Autodesk Inventor part; units mm, degrees
ref_plane "YZ Plane" through (0, 0, 0) normal (1, 0, 0) x (0, 1, 0)
ref_plane "XZ Plane" through (0, 0, 0) normal (0, 1, 0) x (-1, 0, 0)
ref_plane "XY Plane" through (0, 0, 0) normal (0, 0, 1) x (1, 0, 0)
sketch "Sketch2" plane through (0, 0, 0) normal (0, 1, 0) x (-1, 0, 0)
  line L0 (1.6384, 12.2587) -> (39.6384, 12.2587)
  line L1 (49.6384, 5.2687) -> (49.6384, -15.7313)
  line L2 (40.6384, -24.2313) -> (0.6384, -24.2313)
  line L3 (-8.3616, -15.7313) -> (-8.3616, 5.2687)
  line L4 (1.6384, 12.2587) -> (39.6384, 12.2587)
  line L5 (20.6384, 12.2587) -> (1.6384, 12.2587)
  line L6 (1.6384, 12.2587) -> (1.6384, 5.2687)
  line L7 (20.6384, 12.2587) -> (39.6384, 12.2587)
  line L8 (39.6384, 12.2587) -> (39.6384, 5.2687)
  circle A0 centre (31.1384, -0.7313) radius 4
  circle A1 centre (31.1384, 6.2687) radius 1.5
  circle A2 centre (24.1384, -0.7313) radius 1.5
  circle A3 centre (31.1384, -7.7313) radius 1.5
  circle A4 centre (38.1384, -0.7313) radius 1.5
  line L9 (31.1384, -0.7313) -> (40.1384, -0.7313) construction
  circle A5 centre (20.6384, -10.7313) radius 4
  circle A6 centre (20.6384, -3.7313) radius 1.5
  circle A7 centre (13.6384, -10.7313) radius 1.5
  circle A8 centre (20.6384, -17.7313) radius 1.5
  circle A9 centre (27.6384, -10.7313) radius 1.5
  line L10 (20.6384, -10.7313) -> (30.6384, -10.7313) construction
  line L11 (20.6384, 0) -> (20.6384, 3.2687)
  circle A10 centre (10.1384, -0.7313) radius 4
  circle A11 centre (10.1384, 6.2687) radius 1.5
  circle A12 centre (17.1384, -0.7313) radius 1.5
  circle A13 centre (10.1384, -7.7313) radius 1.5
  circle A14 centre (3.1384, -0.7313) radius 1.5
  line L12 (10.1384, -0.7313) -> (1.1384, -0.7313) construction
  line L13 (1.6384, 5.2687) -> (1.6384, 1.7687)
  line L14 (1.6384, 1.7687) -> (0.6384, 1.7687)
  line L15 (0.6384, 1.7687) -> (0.6384, 5.2687)
  line L16 (39.6384, 5.2687) -> (39.6384, 1.7687)
  line L17 (39.6384, 1.7687) -> (40.6384, 1.7687)
  line L18 (40.6384, 1.7687) -> (40.6384, 5.2687)
  circle A15 centre (-3.8616, -1.2313) radius 2
  circle A16 centre (-3.8616, -11.2313) radius 2
  line L19 (0.6384, 5.2687) -> (0.6384, 6.2687)
  line L20 (0.6384, 6.2687) -> (-8.3616, 6.2687)
  line L21 (-8.3616, 6.2687) -> (-8.3616, 5.2687)
  line L22 (40.6384, 5.2687) -> (40.6384, 6.2687)
  line L23 (40.6384, 6.2687) -> (49.6384, 6.2687)
  line L24 (49.6384, 6.2687) -> (49.6384, 5.2687)
  circle A17 centre (45.1384, -1.2313) radius 2
  circle A18 centre (45.1384, -11.2313) radius 2
  line L25 (0.6384, -24.2313) -> (0.6384, -17.7313)
  line L26 (0.6384, -17.7313) -> (-6.3616, -17.7313)
  line L27 (40.6384, -24.2313) -> (40.6384, -17.7313)
  line L28 (40.6384, -17.7313) -> (47.6384, -17.7313)
  arc A19 (-8.3616, -15.7313) -> (-6.3616, -17.7313) centre (-6.3616, -15.7313) ccw
  arc A20 (47.6384, -17.7313) -> (49.6384, -15.7313) centre (47.6384, -15.7313) ccw
  line L29 (1.6384, 12.2587) -> (39.6384, 12.2587)
  line L30 (40.6384, -24.2313) -> (1.6384, -24.2313)
  line L31 (1.6384, 1.7687) -> (1.6384, 12.2587)
  line L32 (40.6384, 6.2687) -> (40.6384, 1.7687)
  line L33 (40.6384, -17.7313) -> (40.6384, -24.2313)
  line L34 (49.6384, 6.2687) -> (49.6384, -15.7313)
  line L35 (-8.3616, -15.7313) -> (-8.3616, 6.2687)
  line L36 (40.6384, 6.2687) -> (49.6384, 6.2687)
  line L37 (-8.3616, 6.2687) -> (0.6384, 6.2687)
  line L38 (47.6384, -17.7313) -> (40.6384, -17.7313)
  line L39 (0.6384, -17.7313) -> (-6.3616, -17.7313)
  line L40 (-8.3616, 6.2687) -> (-8.3616, -15.7313)
  line L41 (-6.3616, -17.7313) -> (0.6384, -17.7313)
  line L42 (0.6384, -24.2313) -> (0.6384, -17.7313)
  line L43 (-6.3616, -17.7313) -> (0.6384, -17.7313)
  line L44 (0.6384, -24.2313) -> (40.6384, -24.2313)
  line L45 (40.6384, -24.2313) -> (40.6384, -17.7313)
  line L46 (40.6384, -17.7313) -> (47.6384, -17.7313)
  line L47 (49.6384, -15.7313) -> (49.6384, 6.2687)
  line L48 (49.6384, 6.2687) -> (40.6384, 6.2687)
  line L49 (40.6384, 6.2687) -> (40.6384, 1.7687)
  line L50 (39.6384, 1.7687) -> (40.6384, 1.7687)
  line L51 (39.6384, 1.7687) -> (39.6384, 12.2587)
  line L52 (39.6384, 12.2587) -> (1.6384, 12.2587)
  line L53 (1.6384, 12.2587) -> (1.6384, 1.7687)
  line L54 (1.6384, 1.7687) -> (0.6384, 1.7687)
  line L55 (0.6384, 1.7687) -> (0.6384, 6.2687)
  line L56 (0.6384, 6.2687) -> (-8.3616, 6.2687)
  line L57 (-8.3616, 6.2687) -> (-8.3616, -15.7313)
  point P0 (0, 0)
  dimension "d12" = 360
  dimension "d19" = 360
  dimension "d22" = 10
  dimension "d23" = 29
  dimension "d24" = 29
  dimension "d25" = 10.5
  dimension "d26" = 21
  dimension "d32" = 1
  dimension "d33" = 3.5
  dimension "d34" = 1
  dimension "d37" = 4
  dimension "d38" = 4
  dimension "d41" = 2
extrude "Extrusion1" add sketch "Sketch2" along normal blind 1
sketch "Sketch3" plane through (0, 1, 0) normal (0, 1, 0) x (1, 0, 0)
  line L0 (-0.6384, 17.7313) -> (-0.6384, 24.2313)
  line L1 (-49.6384, 15.7313) -> (-49.6384, -6.2687)
  line L2 (-0.6384, -1.7687) -> (-0.6384, -6.2687)
  line L3 (8.3616, -6.2687) -> (8.3616, 15.7313)
  line L4 (-40.6384, 24.2313) -> (-0.6384, 24.2313)
  line L5 (-0.6384, 24.2313) -> (-0.6384, 23.2313)
  line L6 (-0.6384, 23.2313) -> (-40.6384, 23.2313)
  line L7 (-40.6384, 23.2313) -> (-40.6384, 24.2313)
  line L8 (-0.6384, -6.2687) -> (8.3616, -6.2687)
  line L9 (8.3616, -6.2687) -> (8.3616, -5.2687)
  line L10 (8.3616, -5.2687) -> (-0.6384, -5.2687)
  line L11 (-40.6384, -6.2687) -> (-49.6384, -6.2687)
  line L12 (-49.6384, -6.2687) -> (-49.6384, -5.2687)
  line L13 (-49.6384, -5.2687) -> (-40.6384, -5.2687)
  line L14 (-40.6384, -5.2687) -> (-40.6384, -6.2687)
  line L15 (-0.6384, -5.2687) -> (-0.6384, -6.2687)
  point P0 (0, 0)
  dimension "d44" = 1
  dimension "d45" = 1
  dimension "d46" = 1
extrude "Extrusion2" add sketch "Sketch3" along normal blind 26
fillet "Fillet1" radius 2 6 edges at (-49.6384, 27, 5.7687) (-40.6384, 27, 5.7687) (8.3616, 27, 5.7687) (-0.6384, 27, 5.7687) (-0.6384, 27, -23.7313) (-40.6384, 27, -23.7313)
sketch "Sketch4" plane through (-40.6384, 1, -23.2313) normal (0, 0, 1) x (1, 0, 0)
  circle A0 centre (10, 12) radius 1.5
  circle A1 centre (10, 5) radius 1.5
  circle A2 centre (17, 12) radius 1.5
  circle A3 centre (10, 19) radius 1.5
  circle A4 centre (3, 12) radius 1.5
  circle A5 centre (30, 12) radius 1.5
  circle A6 centre (30, 5) radius 1.5
  circle A7 centre (37, 12) radius 1.5
  circle A8 centre (30, 19) radius 1.5
  circle A9 centre (23, 12) radius 1.5
  point P0 (40.6384, -1)
  dimension "d52" = 3
  dimension "d55" = 360
  dimension "d58" = 3
  dimension "d59" = 3
  dimension "d62" = 360
extrude "Extrusion3" cut sketch "Sketch4" against normal blind 26
sketch "Sketch5" plane through (-49.6384, 0, 6.2687) normal (0, 0, 1) x (1, 0, 0)
  circle A0 centre (4.5, 19.75) radius 1.5
  circle A1 centre (4.5, 5.25) radius 1.5
  line L0 (2, 27) -> (7, 27)
  line L1 (0, 0) -> (0, 25)
  line L2 (4.5, 27) -> (4.5, 12.5)
  point P0 (49.6384, 0)
  dimension "d66" = 3
  dimension "d69" = 14.5
  dimension "d70" = 7.25
  dimension "d71" = 3
extrude "Extrusion4" cut sketch "Sketch5" against normal blind 26
sketch "Sketch6" plane through (-0.6384, 0, 6.2687) normal (0, 0, 1) x (1, 0, 0)
  circle A0 centre (4.5, 19.75) radius 1.5
  circle A1 centre (4.5, 6.25) radius 1.5
  point P0 (0.6384, 0)
  dimension "d72" = 3
  dimension "d73" = 3
extrude "Extrusion5" cut sketch "Sketch6" against normal blind 26
properties part number "modelo 2"
Build history of the part. All positions in model axes, mm. A direction names the side the tool comes from. Coordinates: 2 decimals unless noted, no trailing zeros. Order: outer loops, then holes, each group sorted by start corner. A loop starts at its lowest first (then second) coordinate and runs counter-clockwise, first axis right, second up. Notation, with made-up numbers: (-14.5, 80) -> (26.5, 80) arc R14 cw to (26.5, 99) -> close; hole circle Ø11 at (44, 49.25). An arc over 180 degrees is marked (long way). One line per item, written item: value.
(1) Tool access for faces 1 (the cylindrical face through (-16.208, 13.451, -23.724)), 2 (the flat face through (-40.638, 11, 6)), 3 (the flat face through (-45, 14, 5.269)): list every direction of +Z, -Z, +X, -X, +Y, -Y with a clear straight run to the whole face (end or side of a thin tool).
Checked values:
face 1: +Z, -Z
face 2: +Z, +Y, -Y
face 3: -Z, +X, -X, +Y
(2) Slice it at C-C, the plane z = -10. List the corners of the cut face in (x, y), plus the area to 3 significant figures.
Checked values:
outline: (-49.64, 0) -> (-46.71, 0) -> (-46.71, 1) -> (-49.64, 1) -> close; (-43.56, 0) -> (-28.95, 0) -> (-28.95, 1) -> (-43.56, 1) -> close; (-26.33, 0) -> (-24.57, 0) -> (-24.57, 1) -> (-26.33, 1) -> close; (-16.71, 0) -> (-14.95, 0) -> (-14.95, 1) -> (-16.71, 1) -> close; (-12.33, 0) -> (2.29, 0) -> (2.29, 1) -> (-12.33, 1) -> close; (5.44, 0) -> (8.36, 0) -> (8.36, 1) -> (5.44, 1) -> close
area: 38.6 mm2
(3) Probe line 1 (Z direction, x = -14, y = 5.75); line 2 (Y direction, x = -43.5, z = -15.5); line 3 (Z direction, x = -46.5, y = 6.25). List the from-to ranges inside material, lowest first. Write a range as [from, to].
Checked values:
line 1: [-24.23, -23.23]
line 2: [0, 1]
line 3: [5.27, 6.27]
(4) Mould opens along X. For faces 4 (the flat face through (-0.638, 10.6, -23.4)), 5 (the flat face through (-20, 0, -6)), 6 (the cylindrical face through (-20.313, 0.493, -2.267)) say: pulls with the +X half, pulls with the -X half, needs draft (parallel to the pull), parting line crosses it, or undercut.
Checked values:
face 4: pulls with the +X half
face 5: needs draft
face 6: undercut
(5) Slice it at A-A, the plane y = 2.5. List the corners of the cut face in (x, z).
Checked values:
outline: (-49.64, 5.27) -> (-40.64, 5.27) -> (-40.64, 6.27) -> (-49.64, 6.27) -> close; (-40.64, -24.23) -> (-0.64, -24.23) -> (-0.64, -23.23) -> (-40.64, -23.23) -> close; (-0.64, 5.27) -> (8.36, 5.27) -> (8.36, 6.27) -> (-0.64, 6.27) -> close
(6) Slice it at D-D, the plane y = 13. Count the separate pieces of the cut face and the enclosed holes in it, plus the area to 3 significant figures.
Checked values:
separate pieces: 9
enclosed holes: 0
area: 40.0 mm2
(7) Slice it at B-B, the plane z = 4. List the corners of the cut face in (x, y).
Checked values:
outline: (-49.64, 0) -> (-40.64, 0) -> (-40.64, 1) -> (-49.64, 1) -> close; (-39.64, 0) -> (-1.64, 0) -> (-1.64, 1) -> (-39.64, 1) -> close; (-0.64, 0) -> (8.36, 0) -> (8.36, 1) -> (-0.64, 1) -> close
(8) Drop flat-ended pins along their axis: pin 1 Ø3 at (x, y) = (-34, 23) entering from +Z; pin 2 Ø10 at (x, y) = (-41, 22.5) entering from +Z; pin 3 Ø8 at (y, z) = (20.5, -20) entering from +X; pin 4 Ø3 at (x, z) = (-5.5, -13.5) entering from -Y. Give the stop position or say it passes through.
Checked values:
pin 1: z = -23.23
pin 2: z = 6.27
pin 3: x = -0.64
pin 4: y = 0
